```python
from build123d import *

# Parameters (mm, degrees)
SKETCH_1_R          = 14.5
EXTRUDE_1_DEPTH     = 5
EXTRUDE_2_DEPTH     = 5
CHAMFER_1_SIZE      = 1
SKETCH_3_R          = 0.85
CUT_EXTRUDE_1_DEPTH = 0.1


with BuildPart() as part:
    # 草图1 → 凸台-拉伸1 (new body)
    with BuildSketch(Plane(origin=(0, 0, 0), x_dir=(0, 0, -1), z_dir=(1, 0, 0))):
        Circle(SKETCH_1_R)
    extrude(amount=EXTRUDE_1_DEPTH)

    # 草图2 → 凸台-拉伸2 (add)
    with BuildSketch(Plane(origin=(5, 0, 0), x_dir=(0, 0, -1), z_dir=(1, 0, 0))):
        with BuildLine():
            ThreePointArc((3, 14.186260959), (1.508180397, 14.421351944), (4.2e-08, 14.5))
            ThreePointArc((4.2e-08, 14.5), (-1.508180355, 14.421351948), (-3, 14.186260959))
            Line((-3, 14.186260959), (-3, -14.186260959))
            ThreePointArc((-3, -14.186260959), (-1.508180376, -14.421351946), (0, -14.5))
            ThreePointArc((0, -14.5), (1.508180376, -14.421351946), (3, -14.186260959))
            Line((3, -14.186260959), (3, 14.186260959))
        make_face()
    extrude(amount=EXTRUDE_2_DEPTH)

    # 倒角1
    chamfer_1_edges = [part.edges().sort_by_distance(p)[0] for p in [
        (10, 14.5, 0),
    ]]
    chamfer(chamfer_1_edges, length=CHAMFER_1_SIZE)

    # 草图3 → 切除-拉伸1 (cut)
    with BuildSketch(Plane(origin=(10, 0, 0), x_dir=(0, 0, -1), z_dir=(1, 0, 0))):
        with Locations((0, 10)):
            Circle(SKETCH_3_R)
    extrude(amount=-CUT_EXTRUDE_1_DEPTH, mode=Mode.SUBTRACT)


solid = part.part
```
Input: part model. Units: mm. Frame: model coordinates. A direction names the side the tool comes from. Round coordinates to 2 decimals unless told otherwise and drop trailing zeros. Loops run counter-clockwise (first coordinate to the right, second up) from the corner with the lowest first, then second, coordinate; pieces in that order, holes last.
1) Section query B-B on x = 8.5. Return the cut outline in (y, z), plus the area to 3 significant figures.
Ans:
outline: (-14.19, -3) - (14.19, -3) arc R14.5 ccw to (14.19, 3) - (-14.19, 3) arc R14.5 ccw to start
area: 173 mm2
2) Section query D-D on z = -12.5. Return the cut outline in (x, y).
Ans:
outline: (0, -7.35) - (5, -7.35) - (5, 7.35) - (0, 7.35) - close
3) Set-up query: faces 1 (the flat face through (5, 0, -7)), 2 (the flat face through (7, 0, 3)), 3 (the flat face through (10, 0, 0)). Return all of +Z, -Z, +X, -X, +Y, -Y with unobstructed straight access to the full face (end or side cutting, diameter ignored); none if empty.
Ans:
face 1: -Z, +X, +Y, -Y
face 2: +Z, +X, +Y, -Y
face 3: +Z, -Z, +X, +Y, -Y
4) Section query A-A on y = 0. Return the cut outline in (x, z).
Ans:
outline: (0, -14.5) - (5, -14.5) - (5, -3) - (10, -3) - (10, 3) - (5, 3) - (5, 14.5) - (0, 14.5) - close
5) Material intervals for line 1 (Z direction, x = 9.75, y = -6); line 2 (X direction, y = -3, z = 6); line 3 (Z direction, x = 4.25, y = 0.25), sorted ascending.
Ans:
line 1: z = -3 to 3
line 2: x = 0 to 5
line 3: z = -14.5 to 14.5
6) Pull-direction query (Y, two-part tool) for faces 4 (the flat face through (5, 0, 8)), 5 (the flat face through (9.9, 10, 0)); classes: released by +Y, released by -Y, zero draft, split by the parting line, or undercut.
Ans:
face 4: zero draft
face 5: undercut
7) Pin query (flat end, axial travel): pin 1 (3 mm diameter, centred on x = 5.5, z = 10, fed in from -Y); pin 2 (1.5 mm diameter, centred on x = 7, y = -5, fed in from -Z); pin 3 (6 mm diameter, centred on y = -0.5, z = 10.5, fed in from +X). Return the tip coordinate at first contact, or that it passes through.
Ans:
pin 1: stops at y = -11.68
pin 2: stops at z = -3
pin 3: stops at x = 5
8) Section query C-C on y = 10. Return the cut outline in (x, z).
Ans:
outline: (0, -10.5) - (5, -10.5) - (5, -3) - (10, -3) - (10, -0.85) - (9.9, -0.85) - (9.9, 0.85) - (10, 0.85) - (10, 3) - (5, 3) - (5, 10.5) - (0, 10.5) - close
